```python
from build123d import *

# Parameters (mm, degrees)
F0_R     = 4.7625
F1_DEPTH = 63.5
F2_SIZE  = 1.27
F4_D     = 3.96875
F4_DEPTH = 60.325
F4_TIP   = 1.1923327909


with BuildPart() as f1:
    # F0 (on Top) → F1 (new body)
    with BuildSketch(Plane.XY):
        Circle(F0_R)
    extrude(amount=F1_DEPTH)

    # F2
    f2_edges = [f1.edges().sort_by_distance(p)[0] for p in [
        (-4.7625, 0, 63.5),
        (-4.7625, 0, 0),
    ]]
    chamfer(f2_edges, length=F2_SIZE)

    # F4
    with Locations(Plane(origin=(0, 0, 0), x_dir=(1, 0, 0), z_dir=(0, 0, -1))):
        with Locations((0, 0)):
            Hole(F4_D / 2, depth=F4_DEPTH)
            with Locations((0, 0, -(F4_DEPTH + F4_TIP / 2))):  # 118° drill point
                Cone(0, F4_D / 2, F4_TIP, mode=Mode.SUBTRACT)


solid = f1.part
```
Check sheet for the modelled part. Datum: model origin and axes. Units: mm. A direction names the side the tool comes from. Round coordinates to 2 decimals unless told otherwise and drop trailing zeros. Loops run counter-clockwise (first coordinate to the right, second up) from the corner with the lowest first, then second, coordinate; pieces in that order, holes last. Notation, with made-up numbers: (18, 61.25) -> (62, 61.25) arc R32 cw to (62, 96.25) -> close; hole circle Ø8 at (-38.5, -25). An arc over 180 degrees is marked (long way). Write item = value, one per line. Start each with the question number.
1) Release check for a two-part mould opening along X. For faces 3 (the cylindrical face through (-3.78, -2.9, 31.32)), 4 (the conical face through (0.33, -0.1, 61.31)), 5 (the flat face through (2, -2, 0)) record: released by +X, released by -X, zero draft, split by the parting line, or undercut.
2) Set-up check for faces 1 (the cylindrical face through (0.43, 1.937, 30.585)), 2 (the flat face through (0, 0, 63.5)): record each of +Z, -Z, +X, -X, +Y, -Y from which the full face is reachable in a straight line by a thin tool's end or side.
3) Thickness scan on probe 1 along Y at (x, z) = (0, 32); probe 2 along X at (y, z) = (-1.5, 38); probe 3 along X at (y, z) = (-1.25, 27). Record the ranges inside material, lowest first.
4) Sectioned sample at A-A, the plane z = 11. Record the cut outline in (x, y) (1 decimal), plus the area to 3 significant figures.
5) Gauge pin test, flat ends, axial feed: pin 1 Ø5 at (x, y) = (-1, -0.5) entering from -Z; pin 2 Ø3 at (x, z) = (2.5, 40) entering from +Y. Record the tip position at first contact, or that the pin passes through.
Results are:
q1.face_3 = split by the parting line
q1.face_4 = undercut
q1.face_5 = zero draft
q2.face_1 = -Z
q2.face_2 = +Z, +X, -X, +Y, -Y
q3.probe_1 = -4.76 to -1.98, 1.98 to 4.76
q3.probe_2 = -4.52 to -1.3, 1.3 to 4.52
q3.probe_3 = -4.6 to -1.54, 1.54 to 4.6
q4.outline = circle Ø9.5 at (0, 0); hole circle Ø4 at (0, 0)
q4.area = 58.9 mm^2
q5.pin_1 = 0
q5.pin_2 = 4.66
